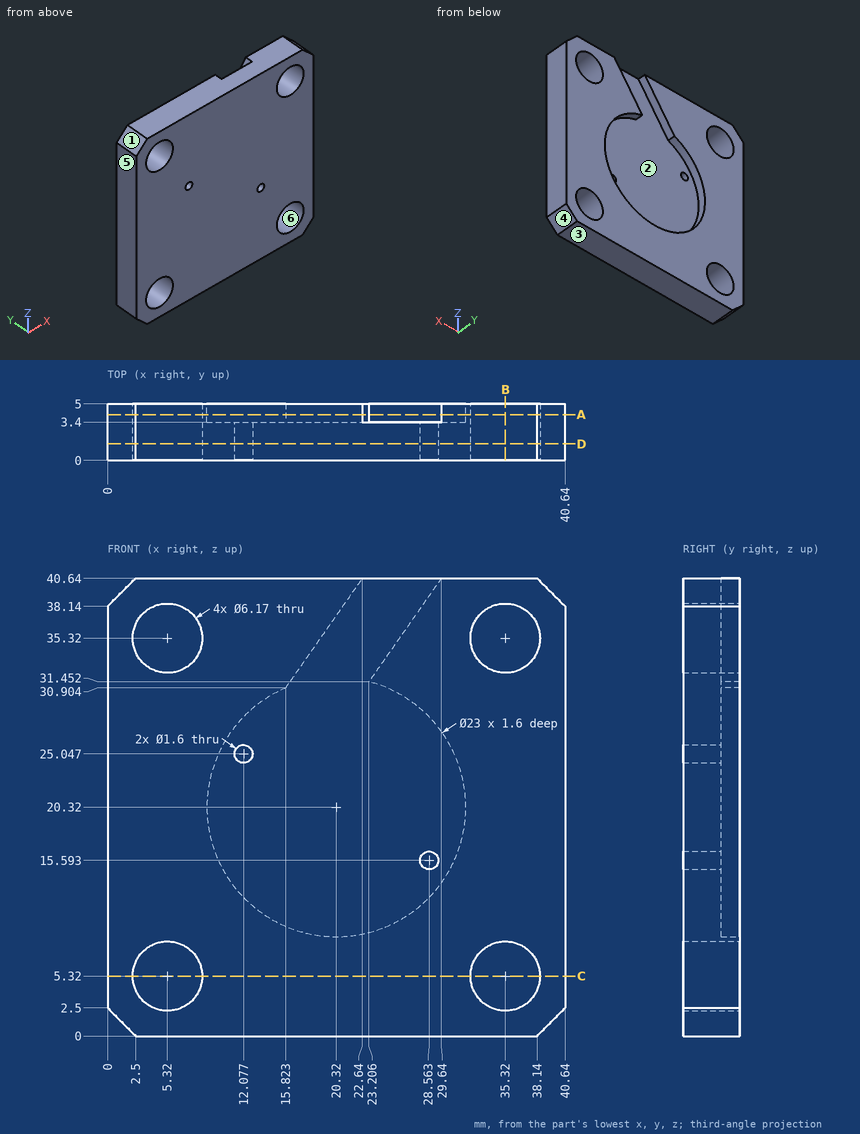
The drawing under review shows one solid part. Ordinate dimensions are in mm from its lowest x, y, z. A direction names the side the tool comes from. Round coordinates to 2 decimals unless told otherwise and drop trailing zeros. Order: outer loops, then holes, each group sorted by start corner. A loop starts at its lowest first (then second) coordinate and runs counter-clockwise, first axis right, second up. Notation, with made-up numbers: (27.5, -12.75) -> (35.5, -12.75) arc R23 ccw to (35.5, 2.25) -> close; hole circle Ø8 at (-24, -10.75). An arc over 180 degrees is marked (long way). Return JSON: item names as keys, results as strings.
1. Take a section at B-B (x = 35.32). Write out the cut boundary in (y, z) (1 decimal).
Answer block:
{"outline": "(0, 0) -> (5, 0) -> (5, 2.2) -> (0, 2.2) -> close; (0, 8.4) -> (5, 8.4) -> (5, 32.2) -> (0, 32.2) -> close; (0, 38.4) -> (5, 38.4) -> (5, 40.6) -> (0, 40.6) -> close"}
2. For the marked faces 1 and 2, list the 3-axis set-ups (+Z, -Z, +X, -X, +Y, -Y) from which the entire face can be reached by the end or side of a thin tool; tool diameter is ignored.
Answer block:
{"face 1": "+Z, -X, +Y, -Y", "face 2": "+Y"}
3. Take a section at D-D (y = 1.45). Write out the cut boundary in (x, z) (1 decimal).
Answer block:
{"outline": "(0, 2.5) -> (2.5, 0) -> (38.1, 0) -> (40.6, 2.5) -> (40.6, 38.1) -> (38.1, 40.6) -> (2.5, 40.6) -> (0, 38.1) -> close; hole circle Ø6.2 at (5.3, 5.3); hole circle Ø6.2 at (5.3, 35.3); hole circle Ø1.6 at (12.1, 25); hole circle Ø1.6 at (28.6, 15.6); hole circle Ø6.2 at (35.3, 5.3); hole circle Ø6.2 at (35.3, 35.3)"}
4. Take a section at A-A (y = 4.05). Write out the cut boundary in (x, z) (1 decimal), then the cut area to 3 significant figures.
Answer block:
{"outline": "(0, 2.5) -> (2.5, 0) -> (38.1, 0) -> (40.6, 2.5) -> (40.6, 38.1) -> (38.1, 40.6) -> (29.6, 40.6) -> (23.2, 31.5) arc R11.5 cw (long way) to (15.8, 30.9) -> (22.6, 40.6) -> (2.5, 40.6) -> (0, 38.1) -> close; hole circle Ø6.2 at (5.3, 5.3); hole circle Ø6.2 at (5.3, 35.3); hole circle Ø6.2 at (35.3, 5.3); hole circle Ø6.2 at (35.3, 35.3)", "area": "1,040 mm²"}
5. For L1, parallel to Z at x = 35.32, y = 1.45 (1 decimal); L2, parallel to Z at x = 3.5, y = 1.9, list the stretches that pass through material, from the lowest coordinate up. Write a range as [from, to].
Answer block:
{"L1": "z = [0, 2.2], [8.4, 32.2], [38.4, 40.6]", "L2": "z = [0, 2.83], [7.81, 32.83], [37.81, 40.64]"}
6. The part is to be moulded in two halves that separate along X. For the marked faces 3, 4, 5 and 6, say which applies: +X half, -X half, draft (parallel to the pull), parting line (faces both ways), or undercut.
Answer block:
{"face 3": "draft", "face 4": "+X half", "face 5": "-X half", "face 6": "undercut"}
7. Take a section at C-C (z = 5.32). Write out the cut boundary in (x, y) (1 decimal).
Answer block:
{"outline": "(0, 0) -> (2.2, 0) -> (2.2, 5) -> (0, 5) -> close; (8.4, 0) -> (32.2, 0) -> (32.2, 5) -> (8.4, 5) -> close; (38.4, 0) -> (40.6, 0) -> (40.6, 5) -> (38.4, 5) -> close"}
8. Insertion check: P1, Ø1.3, axis at x = 28.56, z = 15.59, coming from the +Y side; P2, Ø2, axis at x = 12.08, z = 25.05, coming from the +Y side. Each pin has a flat end and moves straight along its axis. Give the tip position at first contact, or say it passes through.
Answer block:
{"P1": "passes through", "P2": "stops at y = 3.4"}
